Model file for the job. Use its own axes, mm. Coordinates: 2 decimals unless noted, no trailing zeros. Loops run counter-clockwise (first coordinate to the right, second up) from the corner with the lowest first, then second, coordinate; pieces in that order, holes last. Notation, with made-up numbers: (-14, 64.5) -> (36, 64.5) arc R22 cw to (36, 96.5) -> close; hole circle Ø11 at (-36, 15.25). An arc over 180 degrees is marked (long way). Use one line per item in the form item = value.
```python
from build123d import *

# Parameters (mm, degrees)
SKETCH_1_R               = 15
DIAMETER30_HEIGHT8_DEPTH = 8
SKETCH_2_W               = 5.192982456
SKETCH_2_H               = 3.508771929
CHARACTER_DEPTH          = 0.1
SKETCH_3_R               = 13.1
SKETCH_3_R_2             = 12.7
INK_RING_DEPTH           = 0.08


with BuildPart() as part:
    # 草图1 → Diameter30_Height8 (new body)
    with BuildSketch(Plane.XY):
        Circle(SKETCH_1_R)
    extrude(amount=-DIAMETER30_HEIGHT8_DEPTH)

    # 草图2 → Character_兵 (add)
    # profile 1 of 3: a face of its own
    with BuildSketch(Plane.XY):
        with BuildLine():
            add(Edge.make_bspline(
                [(5.385964912, 5.675438596), (5.427646333, 5.544154901), (5.514415642, 5.270858182), (5.718534697, 4.870645294), (5.979105034, 4.460896452), (6.189038604, 4.198106369), (6.298245614, 4.061403509)],
                knots=[0, 0, 0, 0, 0.883893952, 1.840025262, 2.876385589, 4, 4, 4, 4], degree=3))
            add(Edge.make_bspline(
                [(6.298245614, 4.061403509), (5.963833471, 4.026716097), (5.279490907, 3.955731615), (4.231500891, 3.847667949), (3.138573287, 3.746554234), (2.199926718, 3.654410468), (1.420771678, 3.589929187), (0.809223667, 3.542341458), (0.175852477, 3.501012073), (-0.480095669, 3.465441213), (-1.157529916, 3.430930645), (-1.857588828, 3.402476855), (-2.579333786, 3.379715375), (-3.06800455, 3.366400533), (-3.315789474, 3.359649123)],
                knots=[0, 0, 0, 0, 1.255148332, 2.568541377, 3.933119286, 5.35274168, 6.089508688, 6.851809632, 7.642688325, 8.45900384, 9.304218247, 10.174988169, 11.074611272, 12, 12, 12, 12], degree=3))
            Line((-3.315789474, 3.359649123), (-3.315789474, 1.043859649))
            Line((-3.315789474, 1.043859649), (3.350877193, 1.043859649))
            add(Edge.make_bspline(
                [(3.350877193, 1.043859649), (3.511157354, 1.043351179), (3.823930109, 1.042358944), (4.282215924, 1.049417071), (4.718886002, 1.053533845), (5.133897674, 1.061104446), (5.526304771, 1.072707016), (5.896383806, 1.080969698), (6.244544047, 1.09823882), (6.469784841, 1.108878558), (6.578947368, 1.114035088)],
                knots=[0, 0, 0, 0, 1.191206585, 2.324535747, 3.406356757, 4.43677056, 5.409393768, 6.324087995, 7.187772401, 8, 8, 8, 8], degree=3))
            Line((6.578947368, 1.114035088), (6.578947368, -0.289473684))
            add(Edge.make_bspline(
                [(6.578947368, -0.289473684), (6.325999471, -0.278216628), (5.805513386, -0.255053199), (5.003105502, -0.23621154), (4.156642469, -0.222539126), (3.577870773, -0.220397737), (3.280701754, -0.219298246)],
                knots=[0, 0, 0, 0, 0.920900528, 1.894919528, 2.91915119, 4, 4, 4, 4], degree=3))
            Line((3.280701754, -0.219298246), (3.280701754, -3.728070175))
            Line((3.280701754, -3.728070175), (5.175438596, -3.728070175))
            add(Edge.make_bspline(
                [(5.175438596, -3.728070175), (5.437087744, -3.726975877), (5.945690026, -3.724848744), (6.687326433, -3.711192023), (7.384937776, -3.692513148), (7.835209995, -3.669167553), (8.052631579, -3.657894737)],
                knots=[0, 0, 0, 0, 1.090812078, 2.120356657, 3.092382303, 4, 4, 4, 4], degree=3))
            Line((8.052631579, -3.657894737), (8.052631579, -5.061403509))
            add(Edge.make_bspline(
                [(8.052631579, -5.061403509), (7.837808318, -5.050169454), (7.399653446, -5.027256405), (6.728050321, -5.008178757), (6.030595105, -4.994576557), (5.556645778, -4.992356355), (5.315789474, -4.99122807)],
                knots=[0, 0, 0, 0, 0.942753637, 1.922846234, 2.944411245, 4, 4, 4, 4], degree=3))
            Line((5.315789474, -4.99122807), (-4.929824561, -4.99122807))
            add(Edge.make_bspline(
                [(-4.929824561, -4.99122807), (-5.221796086, -4.992303015), (-5.783243216, -4.994370081), (-6.589858446, -5.007824944), (-7.327331729, -5.026367125), (-7.794924107, -5.050102938), (-8.01754386, -5.061403509)],
                knots=[0, 0, 0, 0, 1.134280796, 2.181167151, 3.134057485, 4, 4, 4, 4], degree=3))
            Line((-8.01754386, -5.061403509), (-8.01754386, -3.657894737))
            add(Edge.make_bspline(
                [(-8.01754386, -3.657894737), (-7.918780668, -3.663109409), (-7.710021339, -3.67413185), (-7.380044631, -3.691202686), (-7.016884144, -3.699292609), (-6.621013356, -3.710966152), (-6.192136611, -3.718460184), (-5.730343207, -3.722568458), (-5.235668056, -3.729595696), (-4.895172776, -3.728589765), (-4.719298246, -3.728070175)],
                knots=[0, 0, 0, 0, 0.719411058, 1.520645164, 2.403271333, 3.3614919, 4.401477414, 5.52328659, 6.720714106, 8, 8, 8, 8], degree=3))
            Line((-4.719298246, -3.728070175), (-4.719298246, 1.535087719))
            add(Edge.make_bspline(
                [(-4.719298246, 1.535087719), (-4.718784553, 1.689303498), (-4.717785992, 1.989081562), (-4.724827935, 2.426573997), (-4.728954195, 2.839853385), (-4.736476359, 3.228877821), (-4.748135548, 3.593555392), (-4.756324903, 3.934194089), (-4.77353537, 4.251158894), (-4.784297949, 4.45473273), (-4.789473684, 4.552631579)],
                knots=[0, 0, 0, 0, 1.226022714, 2.383249742, 3.478491498, 4.511863319, 5.476544353, 6.379262498, 7.220585815, 8, 8, 8, 8], degree=3))
            add(Edge.make_bspline(
                [(-4.789473684, 4.552631579), (-4.268706026, 4.556028892), (-3.23884814, 4.562747339), (-1.711781979, 4.634250298), (-0.219866652, 4.740633472), (0.993183313, 4.869797657), (1.923704926, 4.988295648), (2.567560235, 5.078693798), (3.161212168, 5.171746835), (3.703352911, 5.268528417), (4.196476895, 5.362226591), (4.637690365, 5.465343924), (5.030740941, 5.563211427), (5.272785841, 5.639681531), (5.385964912, 5.675438596)],
                knots=[0, 0, 0, 0, 1.826039719, 3.611133242, 5.359645429, 7.070379028, 7.888093123, 8.64899991, 9.350260421, 9.995089588, 10.580183652, 11.110071571, 11.583873602, 12, 12, 12, 12], degree=3))
        make_face()
        with Locations((-0.719298246, -1.973684211)):
            Rectangle(SKETCH_2_W, SKETCH_2_H, mode=Mode.SUBTRACT)
    # profile 2 of 3: a face of its own
    with BuildSketch(Plane.XY):
        with BuildLine():
            add(Edge.make_bspline(
                [(-2.122807018, -6.254385965), (-2.157477947, -6.282955909), (-2.239146675, -6.350253527), (-2.380099943, -6.467370774), (-2.555580621, -6.61772706), (-2.766181537, -6.799581185), (-3.010546273, -7.013645708), (-3.292157091, -7.257784349), (-3.608078345, -7.535369573), (-4.067550245, -7.940488445), (-4.641654961, -8.448307776), (-5.298106508, -9.038691618), (-5.905984263, -9.586353364), (-6.289571124, -9.942900475), (-6.473684211, -10.114035088)],
                knots=[0, 0, 0, 0, 0.2780539, 0.654966813, 1.134206325, 1.708249881, 2.37711475, 3.1448483, 4.014977533, 4.979944052, 6.936134783, 8.758754283, 10.444274784, 12, 12, 12, 12], degree=3))
            add(Edge.make_bspline(
                [(-6.473684211, -10.114035088), (-6.56675088, -10.003646022), (-6.746034395, -9.790992666), (-7.041333181, -9.517105251), (-7.343912266, -9.291855461), (-7.560952619, -9.184075455), (-7.666666667, -9.131578947)],
                knots=[0, 0, 0, 0, 1.110089453, 2.138474913, 3.093305237, 4, 4, 4, 4], degree=3))
            add(Edge.make_bspline(
                [(-7.666666667, -9.131578947), (-7.459526486, -8.969004344), (-7.051586638, -8.648831509), (-6.464306615, -8.155016872), (-5.902342388, -7.666058703), (-5.371814437, -7.172889256), (-4.86718458, -6.682628792), (-4.391277213, -6.192029207), (-3.945527473, -5.699881064), (-3.664825977, -5.366338586), (-3.526315789, -5.201754386)],
                knots=[0, 0, 0, 0, 1.104789882, 2.175762404, 3.219109849, 4.230036466, 5.214606813, 6.170942573, 7.097464421, 8, 8, 8, 8], degree=3))
            add(Edge.make_bspline(
                [(-3.526315789, -5.201754386), (-3.402072492, -5.313438732), (-3.163971761, -5.527471401), (-2.800509792, -5.808406095), (-2.461726053, -6.055622784), (-2.232199656, -6.190231325), (-2.122807018, -6.254385965)],
                knots=[0, 0, 0, 0, 1.1399807, 2.184667066, 3.134809496, 4, 4, 4, 4], degree=3))
        make_face()
    # profile 3 of 3: a face of its own
    with BuildSketch(Plane.XY):
        with BuildLine():
            add(Edge.make_bspline(
                [(3.49122807, -5.131578947), (3.64506879, -5.27574038), (3.958953573, -5.569876289), (4.429694762, -6.029809869), (4.906171195, -6.5186042), (5.550446937, -7.196959293), (6.333416052, -8.059114332), (6.921508711, -8.778189908), (7.210526316, -9.131578947)],
                knots=[0, 0, 0, 0, 0.694198963, 1.416390223, 2.166820141, 2.941675304, 4.4969891, 6, 6, 6, 6], degree=3))
            add(Edge.make_bspline(
                [(7.210526316, -9.131578947), (7.075068051, -9.202301891), (6.810022921, -9.340682313), (6.440864575, -9.578307626), (6.104530191, -9.83226378), (5.905037831, -10.021201035), (5.807017544, -10.114035088)],
                knots=[0, 0, 0, 0, 1.065427554, 2.08467446, 3.058907518, 4, 4, 4, 4], degree=3))
            add(Edge.make_bspline(
                [(5.807017544, -10.114035088), (5.775308721, -10.061834257), (5.708542231, -9.951919541), (5.596075389, -9.783319805), (5.468667601, -9.601351476), (5.325294262, -9.406676418), (5.167099041, -9.197729098), (4.988610452, -8.978683169), (4.801321577, -8.740479229), (4.591580283, -8.495595111), (4.370378942, -8.233593029), (4.132600709, -7.959359408), (3.876016732, -7.67337978), (3.606767352, -7.371008487), (3.318813913, -7.058440113), (3.015682826, -6.732539485), (2.699522295, -6.391233684), (2.480469315, -6.161414802), (2.368421053, -6.043859649)],
                knots=[0, 0, 0, 0, 0.549342762, 1.156702925, 1.82258923, 2.54738719, 3.331395419, 4.179695988, 5.088851071, 6.056731025, 7.079525855, 8.173336188, 9.321433762, 10.535553977, 11.815185591, 13.144150694, 14.539198359, 16, 16, 16, 16], degree=3))
            add(Edge.make_bspline(
                [(2.368421053, -6.043859649), (2.471264109, -5.972803187), (2.674770245, -5.832196455), (2.965216422, -5.609367892), (3.237954519, -5.37712719), (3.407172595, -5.213070577), (3.49122807, -5.131578947)],
                knots=[0, 0, 0, 0, 1.035169059, 2.048395507, 3.030582027, 4, 4, 4, 4], degree=3))
        make_face()
    extrude(amount=CHARACTER_DEPTH)

    # 草图3 → Ink_ring (add)
    with BuildSketch(Plane.XY):
        with Locations(Location((0, 0, 0), (0, 0, 180))):
            Circle(SKETCH_3_R)
        with Locations(Location((0, 0, 0), (0, 0, 180))):
            Circle(SKETCH_3_R_2, mode=Mode.SUBTRACT)
    extrude(amount=INK_RING_DEPTH)


solid = part.part
```
Q1. Pin check, flat tips, straight feed: pin 1 Ø1 at (x, z) = (-5, -2.5) entering from -Y; pin 2 Ø2 at (x, z) = (-9.5, -7) entering from +Y. Stop position of each tip, or through.
Result:
pin_1 = -14.31
pin_2 = 12.36
Q2. Wall check: line 1 along Z through (x, y) = (-0.25, 12); line 2 along Z through (x, y) = (-7.25, -10.75); line 3 along Y through (x, z) = (5.25, -1.25). Give the ranges that are in metal, low to high.
Result:
line_1 = -8 to 0
line_2 = -8 to 0.08
line_3 = -14.05 to 14.05
Q3. Band-saw the part on A-A, the plane y = -2.5. Write the cut outline in (x, z).
Result:
outline = (-14.79, -8) -> (14.79, -8) -> (14.79, 0) -> (12.86, 0) -> (12.86, 0.08) -> (12.45, 0.08) -> (12.45, 0) -> (3.28, 0) -> (3.28, 0.1) -> (1.88, 0.1) -> (1.88, 0) -> (-3.32, 0) -> (-3.32, 0.1) -> (-4.72, 0.1) -> (-4.72, 0) -> (-12.45, 0) -> (-12.45, 0.08) -> (-12.86, 0.08) -> (-12.86, 0) -> (-14.79, 0) -> close
Q4. Band-saw the part on D-D, the plane y = 9.5. Write the cut outline in (x, z).
Result:
outline = (-11.61, -8) -> (11.61, -8) -> (11.61, 0) -> (9.02, 0) -> (9.02, 0.08) -> (8.43, 0.08) -> (8.43, 0) -> (-8.43, 0) -> (-8.43, 0.08) -> (-9.02, 0.08) -> (-9.02, 0) -> (-11.61, 0) -> close
Q5. Mould opens along Y. For faces 1 (the face through (0, 3, 0)), 2 (the face through (-14.985, 0.66, -3.944)), 3 (the face through (0, 0, -8)) say: released by +Y, released by -Y, zero draft, split by the parting line, or undercut.
Result:
face_1 = undercut
face_2 = split by the parting line
face_3 = zero draft
Q6. Band-saw the part on B-B, the plane z = -7. Write the cut outline in (x, y).
Result:
outline = circle Ø30 at (0, 0)
Q7. Band-saw the part on C-C, the plane x = -10.5. Write the cut outline in (y, z).
Result:
outline = (-10.71, -8) -> (10.71, -8) -> (10.71, 0) -> (7.83, 0) -> (7.83, 0.08) -> (7.14, 0.08) -> (7.14, 0) -> (-7.14, 0) -> (-7.14, 0.08) -> (-7.83, 0.08) -> (-7.83, 0) -> (-10.71, 0) -> close
